Model file for the job. Use its own axes, mm. Face numbers are marked on the shaded views. A direction names the side the tool comes from. Coordinates: 2 decimals unless noted, no trailing zeros. Write each loop counter-clockwise with the first axis right and the second up, starting at its lowest first coordinate (ties: lowest second). Pieces come first, ordered by that corner, then holes. Notation, with made-up numbers: M -37.75,4.25 L -31.75,4.25 A16 cw -31.75,22.25 Z; hole C 65,36.5 d2. An arc over 180 degrees is marked long. Answer in a Markdown table with one row per item. Add a question column.
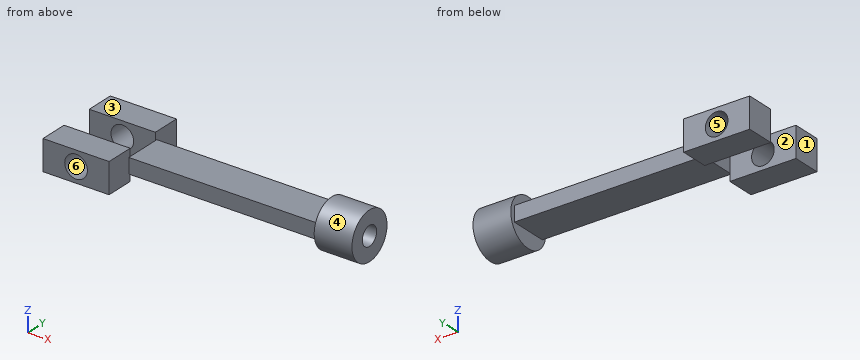
```python
from build123d import *

# Parameters (mm, degrees)
ESQUISSE1_W                  = 100
ESQUISSE1_H                  = 20
BOSS_EXTRU_1_DEPTH           = 4
BOSS_EXTRU_2_DEPTH           = 4
BOSS_EXTRU_2_DEPTH_BACK      = 12
ESQUISSE2_W                  = 35
ESQUISSE2_H                  = 48
ENL_V_MAT_EXTRU_1_DEPTH      = 90.134729483
ENL_V_MAT_EXTRU_1_DEPTH_BACK = 90.134729483
ESQUISSE3_W                  = 35
ESQUISSE3_H                  = 18
ENL_V_MAT_EXTRU_2_DEPTH      = 98.943861472
ENL_V_MAT_EXTRU_2_DEPTH_BACK = 98.943861472
ESQUISSE6_R                  = 6
ESQUISSE7_R                  = 12.5
BOSS_EXTRU_3_DEPTH           = 20
M12_TAPPED_HOLE1_D           = 10.2
M12_TAPPED_HOLE1_DEPTH       = 18
M12_TAPPED_HOLE1_TIP         = 3.064389157


with BuildPart() as part:
    # Esquisse1 → Boss.-Extru.1 (new, symmetric)
    with BuildSketch(Plane.XY):
        Rectangle(ESQUISSE1_W, ESQUISSE1_H)
    extrude(amount=BOSS_EXTRU_1_DEPTH, both=True)

    # Esquisse2 → Boss.-Extru.2 (add, two sides: drawn at the far end of the back side and taken through both)
    with BuildSketch(Plane.XY.offset(4).offset(-BOSS_EXTRU_2_DEPTH_BACK)):
        with Locations((-67.5, 0)):
            Rectangle(ESQUISSE2_W, ESQUISSE2_H)
    extrude(amount=BOSS_EXTRU_2_DEPTH + BOSS_EXTRU_2_DEPTH_BACK)

    # Esquisse3 → Enl_v. mat.-Extru.1 (cut, two sides: drawn at the far end of the back side and taken through both)
    with BuildSketch(Plane.XY.offset(4).offset(-ENL_V_MAT_EXTRU_1_DEPTH_BACK)):
        with Locations((-67.5, 0)):
            Rectangle(ESQUISSE3_W, ESQUISSE3_H)
    extrude(amount=ENL_V_MAT_EXTRU_1_DEPTH + ENL_V_MAT_EXTRU_1_DEPTH_BACK, mode=Mode.SUBTRACT)

    # Esquisse6 → Enl_v. mat.-Extru.2 (cut, two sides: drawn at the far end of the back side and taken through both)
    with BuildSketch(Plane(origin=(0, 24, 0), x_dir=(1, 0, 0), z_dir=(0, 1, 0)).offset(-ENL_V_MAT_EXTRU_2_DEPTH_BACK)):
        with Locations(Location((-67.5, 0, 0), (0, 0, 180))):
            Circle(ESQUISSE6_R)
    extrude(amount=ENL_V_MAT_EXTRU_2_DEPTH + ENL_V_MAT_EXTRU_2_DEPTH_BACK, mode=Mode.SUBTRACT)

    # Esquisse7 → Boss.-Extru.3 (add)
    with BuildSketch(Plane(origin=(50, 0, 0), x_dir=(0, 0, -1), z_dir=(1, 0, 0))):
        Circle(ESQUISSE7_R)
    extrude(amount=BOSS_EXTRU_3_DEPTH)

    # M12 Tapped Hole1
    with Locations(Plane(origin=(70, 0, 0), x_dir=(0, 0, -1), z_dir=(1, 0, 0))):
        with Locations((0, 0)):
            Hole(M12_TAPPED_HOLE1_D / 2, depth=M12_TAPPED_HOLE1_DEPTH)
            with Locations((0, 0, -(M12_TAPPED_HOLE1_DEPTH + M12_TAPPED_HOLE1_TIP / 2))):  # 118° drill point
                Cone(0, M12_TAPPED_HOLE1_D / 2, M12_TAPPED_HOLE1_TIP, mode=Mode.SUBTRACT)


solid = part.part
```
1) Two-plate mould, pull along Z, no slides. Class the marked faces 3, 4, 5 and 6: released by +Z, released by -Z, zero draft, split by the parting line, or undercut.
2) Slice it at A-A (x = -67.5). Give the cut face in (y, z), then the cut area to 3 significant figures.
3) Slice it at B-B (y = 7.5). Give the cut face in (x, z).
4) Drill centre lines: probe 1 along X at (y, z) = (-10.5, -1); probe 2 along Y at (x, z) = (-77, -2); probe 3 along X at (y, z) = (-13.5, 0). Where is each one in solid material? Low to high.
5) Flat gauge pins, fed straight in: pin 1 Ø3 at (x, y) = (-30, 3.5) entering from +Z; pin 2 Ø1.5 at (x, y) = (-61.5, -11) entering from -Z; pin 3 Ø4 at (x, y) = (33, -12.5) entering from +Z; pin 4 Ø4 at (y, z) = (-1, -0.5) entering from -X. Where does each tip first touch, or does it go through?
6) Which spindle directions (+Z, -Z, +X, -X, +Y, -Y) get a long thin tool onto all of the face, cutting with end or side? Do the marked faces 1 and 2. Say none if no direction does.
7) Slice it at C-C (y = 15). Give the cut face in (x, z), then the cut area to 3 significant figures.
8) Slice it at D-D (x = 31). Give the cut face in (y, z).
Ans:
| question | item | result |
|---|---|---|
| 1 | face 3 | released by +Z |
| 1 | face 4 | split by the parting line |
| 1 | face 5 | undercut |
| 1 | face 6 | undercut |
| 2 | outline | M -24,-8 L -9,-8 L -9,-6 L -24,-6 Z; M -24,6 L -9,6 L -9,8 L -24,8 Z; M 9,-8 L 24,-8 L 24,-6 L 9,-6 Z; M 9,6 L 24,6 L 24,8 L 9,8 Z |
| 2 | area | 120 mm2 |
| 3 | outline | M -50,-4 L 50,-4 L 50,-10 L 70,-10 L 70,10 L 50,10 L 50,4 L -50,4 Z |
| 4 | probe 1 | x = -85 to -73.42, -61.58 to -50, 50 to 70 |
| 4 | probe 2 | y = -24 to -9, 9 to 24 |
| 4 | probe 3 | x = -85 to -73.5, -61.5 to -50 |
| 5 | pin 1 | stops at z = 4 |
| 5 | pin 2 | stops at z = -8 |
| 5 | pin 3 | passes through |
| 5 | pin 4 | stops at x = -50 |
| 6 | face 1 | +Z, -Z, -X, +Y, -Y |
| 6 | face 2 | +Z, -Z, -X |
| 7 | outline | M -85,-8 L -50,-8 L -50,8 L -85,8 Z; hole C -67.5,0 d12 |
| 7 | area | 447 mm2 |
| 8 | outline | M -10,-4 L 10,-4 L 10,4 L -10,4 Z |
